```python
from build123d import *

# Parameters (mm, degrees)
PAD004_DEPTH             = 0.3
SKETCH003_W              = 0.25
SKETCH003_H              = 2.4
SKETCH003_H_2            = 1.9
PAD011_DEPTH             = 0.05
SKETCH003_MIRRORED_2_W   = 0.25
SKETCH003_MIRRORED_2_H   = 2.4
SKETCH003_MIRRORED_2_H_2 = 1.9
PAD011_MIRRORED_2_DEPTH  = 0.05
CHAMFER_SIZE             = 0.15
FILLET_R                 = 0.15


with BuildPart() as part:
    # Sketch001 → Pad004 (new body, symmetric)
    with BuildSketch(Plane.XY):
        with BuildLine():
            Line((3.445, 1.7), (3.445, 0))
            Line((3.445, 0), (-3.445, 0))
            Line((-3.445, 0), (-3.445, 1.7))
            ThreePointArc((-3.445, 1.7), (-3.232868, 1.787868), (-3.145, 2))
            Line((-3.145, 2), (-3.145, 2.9))
            ThreePointArc((-3.145, 2.9), (-3.232868, 3.112132), (-3.445, 3.2))
            Line((-3.445, 3.7), (-3.445, 3.2))
            Line((-3.195, 4.45), (-3.445, 3.7))
            Line((-3.195, 4.45), (3.195, 4.45))
            Line((3.195, 4.45), (3.445, 3.7))
            Line((3.445, 3.7), (3.445, 3.2))
            ThreePointArc((3.445, 3.2), (3.232868, 3.112132), (3.145, 2.9))
            Line((3.145, 2.9), (3.145, 2))
            ThreePointArc((3.145, 2), (3.232868, 1.787868), (3.445, 1.7))
        make_face()
    extrude(amount=PAD004_DEPTH, both=True)

    # Sketch003 (on Face16 of Pad004) → Pad011 (join)
    with BuildSketch(Plane.XY.offset(0.3)):
        with Locations((-2.75, 2.8)):
            Rectangle(SKETCH003_W, SKETCH003_H)
        with Locations((-1.25, 2.8)):
            Rectangle(SKETCH003_W, SKETCH003_H)
        with Locations((-2.25, 2.55)):
            Rectangle(SKETCH003_W, SKETCH003_H_2)
        with Locations((-1.75, 2.55)):
            Rectangle(SKETCH003_W, SKETCH003_H_2)
        with Locations((-0.75, 2.55)):
            Rectangle(SKETCH003_W, SKETCH003_H_2)
        with Locations((-0.25, 2.55)):
            Rectangle(SKETCH003_W, SKETCH003_H_2)
    pad011 = extrude(amount=PAD011_DEPTH)

    # Sketch003 Mirrored 2 → Pad011 Mirrored 2 (add)
    with BuildSketch(Plane(origin=(0, 0, 0.3), x_dir=(-1, 0, 0), z_dir=(0, 0, -1))):
        with Locations((-2.75, 2.8)):
            Rectangle(SKETCH003_MIRRORED_2_W, SKETCH003_MIRRORED_2_H)
        with Locations((-1.25, 2.8)):
            Rectangle(SKETCH003_MIRRORED_2_W, SKETCH003_MIRRORED_2_H)
        with Locations((-2.25, 2.55)):
            Rectangle(SKETCH003_MIRRORED_2_W, SKETCH003_MIRRORED_2_H_2)
        with Locations((-1.75, 2.55)):
            Rectangle(SKETCH003_MIRRORED_2_W, SKETCH003_MIRRORED_2_H_2)
        with Locations((-0.75, 2.55)):
            Rectangle(SKETCH003_MIRRORED_2_W, SKETCH003_MIRRORED_2_H_2)
        with Locations((-0.25, 2.55)):
            Rectangle(SKETCH003_MIRRORED_2_W, SKETCH003_MIRRORED_2_H_2)
    pad011_mirrored_2 = extrude(amount=-PAD011_MIRRORED_2_DEPTH)

    # Mirrored001: Pad011, Pad011 Mirrored 2 across XY
    add(pad011.mirror(Plane.XY))
    add(pad011_mirrored_2.mirror(Plane.XY))

    # Chamfer
    chamfer_edges = [part.edges().sort_by_distance(p)[0] for p in [
        (0, 4.45, -0.3),
        (0, 4.45, 0.3),
    ]]
    chamfer(chamfer_edges, length=CHAMFER_SIZE)

    # Fillet
    fillet_edges = [part.edges().sort_by_distance(p)[0] for p in [
        (-3.445, 3.45, 0.3),
        (-3.445, 3.45, -0.3),
        (-3.445, 0.85, 0.3),
        (-3.445, 0.85, -0.3),
        (3.445, 0.85, 0.3),
        (3.445, 0.85, -0.3),
        (3.445, 3.45, 0.3),
        (3.445, 3.45, -0.3),
    ]]
    fillet(fillet_edges, radius=FILLET_R)


solid = part.part
```
The listing builds one solid part. Answer for the finished solid, in the listing's coordinates (mm). Round coordinates to 2 decimals unless told otherwise and drop trailing zeros. Write each loop counter-clockwise with the first axis right and the second up, starting at its lowest first coordinate (ties: lowest second). Pieces come first, ordered by that corner, then holes. Notation, with made-up numbers: (77.5, 15.5) -> (102.5, 15.5) arc R25 ccw to (102.5, 31.5) -> close; hole circle Ø9 at (18, 41.5). An arc over 180 degrees is marked (long way). Use CSV: the item, a comma, the result in double quotes. Start each with the question number.
(1) Section A-A on z = 0.05 is taken. Give the vertices of the cut face in (x, y) (3 decimals).
(2) Section B-B on x = 1.25 is taken. Give the vertices of the cut face in (y, z).
(3) Consider L1, parallel to Z at x = -1, y = 1.3; L2, parallel to X at y = 2.05, z = 0.25 (3 decimals); L3, parallel to X at y = 1, z = 0.2. Determine where each line is inside the solid, lowest interval first. Write a range as from..to.
(4) This flat-tipped pin is pushed along its axis until it touches: pin 1 (1 mm diameter, centred on x = -1.5, y = 1, fed in from +Z). Where does it stop, or does it pass through?
(5) Section C-C on y = 1.2 is taken. Give the vertices of the cut face in (x, z) (3 decimals).
A:
1,outline,"(-3.445, 0) -> (3.445, 0) -> (3.445, 1.7) arc R0.3 cw to (3.145, 2) -> (3.145, 2.9) arc R0.3 cw to (3.445, 3.2) -> (3.445, 3.7) -> (3.195, 4.45) -> (-3.195, 4.45) -> (-3.445, 3.7) -> (-3.445, 3.2) arc R0.3 cw to (-3.145, 2.9) -> (-3.145, 2) arc R0.3 cw to (-3.445, 1.7) -> close"
2,outline,"(0, -0.3) -> (1.6, -0.3) -> (1.6, -0.35) -> (4, -0.35) -> (4, -0.3) -> (4.3, -0.3) -> (4.45, -0.15) -> (4.45, 0.15) -> (4.3, 0.3) -> (4, 0.3) -> (4, 0.35) -> (1.6, 0.35) -> (1.6, 0.3) -> (0, 0.3) -> close"
3,L1,"z = -0.3..0.3"
3,L2,"x = -3.145..3.145"
3,L3,"x = -3.44..3.44"
4,pin 1,"stops at z = 0.3"
5,outline,"(-3.445, -0.15) arc R0.15 ccw to (-3.295, -0.3) -> (3.295, -0.3) arc R0.15 ccw to (3.445, -0.15) -> (3.445, 0.15) arc R0.15 ccw to (3.295, 0.3) -> (-3.295, 0.3) arc R0.15 ccw to (-3.445, 0.15) -> close"
